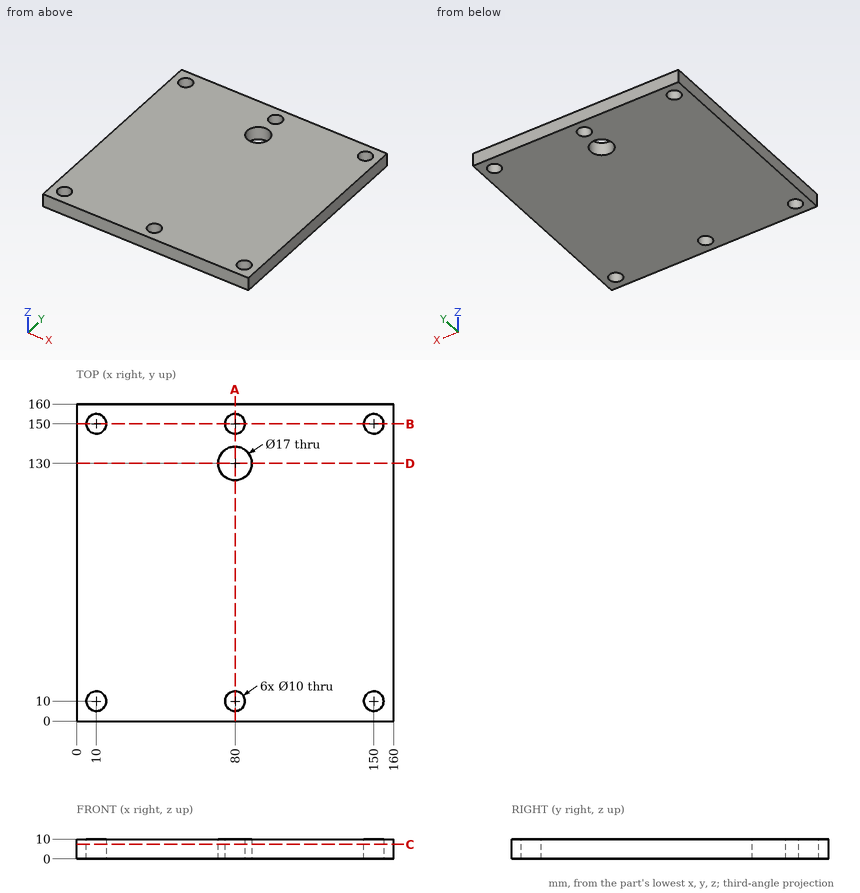
Could you check a few things on this drawing? It's one solid part, dimensions in mm from its lowest x, y, z. Round coordinates to 2 decimals unless told otherwise and drop trailing zeros. Order: outer loops, then holes, each group sorted by start corner. A loop starts at its lowest first (then second) coordinate and runs counter-clockwise, first axis right, second up. Notation, with made-up numbers: M -14.5,53.25 L 21.5,53.25 A23 ccw 21.5,80.25 Z; hole C -34.75,31 d5. An arc over 180 degrees is marked long. Return JSON: item names as keys, results as strings. Group by question number.
1. I'm going to push a flat-ended pin straight in: pin 1 Ø10 at (x, y) = (112.5, 60) entering from -Z. Where does the tip first touch, or does it pass through?
2. If we section it at B-B on y = 150: List the corners of the cut face in (x, z) for me.
3. If we section it at C-C on z = 7.25: List the corners of the cut face in (x, y) for me.
4. If we section it at A-A on x = 80: List the corners of the cut face in (y, z) for me.
5. If we section it at D-D on y = 130: List the corners of the cut face in (x, z) for me, then the cut area to 3 significant figures.
6. Please list where these lines run through material, in increasing order: probe 1 along Y at (x, z) = (80, 7.25); probe 2 along Y at (x, z) = (150, 3.75); probe 3 along X at (y, z) = (150, 7).
Reply:
{
 "1": {"pin 1": "z = 0"},
 "2": {"outline": "M 0,0 L 5,0 L 5,10 L 0,10 Z; M 15,0 L 75,0 L 75,10 L 15,10 Z; M 85,0 L 145,0 L 145,10 L 85,10 Z; M 155,0 L 160,0 L 160,10 L 155,10 Z"},
 "3": {"outline": "M 0,0 L 160,0 L 160,160 L 0,160 Z; hole C 10,10 d10; hole C 10,150 d10; hole C 80,130 d17; hole C 80,10 d10; hole C 80,150 d10; hole C 150,10 d10; hole C 150,150 d10"},
 "4": {"outline": "M 0,0 L 5,0 L 5,10 L 0,10 Z; M 15,0 L 121.5,0 L 121.5,10 L 15,10 Z; M 138.5,0 L 145,0 L 145,10 L 138.5,10 Z; M 155,0 L 160,0 L 160,10 L 155,10 Z"},
 "5": {"outline": "M 0,0 L 71.5,0 L 71.5,10 L 0,10 Z; M 88.5,0 L 160,0 L 160,10 L 88.5,10 Z", "area": "1,430 mm^2"},
 "6": {"probe 1": "0 to 5, 15 to 121.5, 138.5 to 145, 155 to 160", "probe 2": "0 to 5, 15 to 145, 155 to 160", "probe 3": "0 to 5, 15 to 75, 85 to 145, 155 to 160"}
}
